Can you work these out from the model? Positions are in its coordinate system, mm. Coordinates: 2 decimals unless noted, no trailing zeros. Loops run counter-clockwise (first coordinate to the right, second up) from the corner with the lowest first, then second, coordinate; pieces in that order, holes last.
```python
from build123d import *

# Parameters (mm, degrees)
SKETCH1_W           = 6
SKETCH1_H           = 50
SKETCH1_W_2         = 50
SKETCH1_H_2         = 6
BOSS_EXTRUDE1_DEPTH = 6


with BuildPart() as part:
    # Sketch1 → Boss-Extrude1 (new body)
    with BuildSketch(Plane(origin=(0, 0, 0), x_dir=(0, 0, -1), z_dir=(1, 0, 0))):
        with BuildLine():
            Line((-396.831767264, 351.151199882), (21.168232736, 351.151199882))
            ThreePointArc((21.168232736, 351.151199882), (91.878910855, 321.861878001), (121.168232736, 251.151199882))
            Line((121.168232736, 251.151199882), (121.168232736, -330.848800118))
            Line((121.168232736, -330.848800118), (-396.831767264, -330.848800118))
            Line((-396.831767264, -330.848800118), (-396.831767264, 351.151199882))
        make_face()
        with Locations((-375.831767264, 251.151199882)):
            Rectangle(SKETCH1_W, SKETCH1_H, mode=Mode.SUBTRACT)
        with Locations((-375.831767264, -230.848800118)):
            Rectangle(SKETCH1_W, SKETCH1_H, mode=Mode.SUBTRACT)
        with Locations((-235.831767264, -309.848800118)):
            Rectangle(SKETCH1_W_2, SKETCH1_H_2, mode=Mode.SUBTRACT)
        with Locations((-39.831767264, -309.848800118)):
            Rectangle(SKETCH1_W_2, SKETCH1_H_2, mode=Mode.SUBTRACT)
        with Locations((-235.831767264, -219.848800118)):
            Rectangle(SKETCH1_W_2, SKETCH1_H_2, mode=Mode.SUBTRACT)
        with Locations((-39.831767264, -219.848800118)):
            Rectangle(SKETCH1_W_2, SKETCH1_H_2, mode=Mode.SUBTRACT)
        with Locations((-235.831767264, -129.848800118)):
            Rectangle(SKETCH1_W_2, SKETCH1_H_2, mode=Mode.SUBTRACT)
        with Locations((-39.831767264, -129.848800118)):
            Rectangle(SKETCH1_W_2, SKETCH1_H_2, mode=Mode.SUBTRACT)
        with Locations((-235.831767264, -39.848800118)):
            Rectangle(SKETCH1_W_2, SKETCH1_H_2, mode=Mode.SUBTRACT)
        with Locations((-39.831767264, -39.848800118)):
            Rectangle(SKETCH1_W_2, SKETCH1_H_2, mode=Mode.SUBTRACT)
        with Locations((-267.331767264, 308.151199882)):
            Rectangle(SKETCH1_W, SKETCH1_H, mode=Mode.SUBTRACT)
        with Locations((-137.831767264, 308.151199882)):
            Rectangle(SKETCH1_W, SKETCH1_H, mode=Mode.SUBTRACT)
    extrude(amount=BOSS_EXTRUDE1_DEPTH)


solid = part.part
```
Item 1: Suppose I cut it at B-B, the plane x = 1. Count the separate pieces of the cut face and the enclosed holes in it, plus the area to 3 significant figures.
Results are:
separate pieces: 1
enclosed holes: 12
area: 348,000 mm2
Item 2: Suppose I cut it at A-A, the plane z = 222.5. Please give me the cut outline in (x, y), plus the area to 3 significant figures.
Results are:
outline: (0, -330.85) - (6, -330.85) - (6, -312.85) - (0, -312.85) - close; (0, -306.85) - (6, -306.85) - (6, -222.85) - (0, -222.85) - close; (0, -216.85) - (6, -216.85) - (6, -132.85) - (0, -132.85) - close; (0, -126.85) - (6, -126.85) - (6, -42.85) - (0, -42.85) - close; (0, -36.85) - (6, -36.85) - (6, 351.15) - (0, 351.15) - close
area: 3,950 mm2
Item 3: I need wall thicknesses on line 1 along Y through (x, z) = (5.4, 34); line 2 along Z through (x, y) = (4.7, 229); line 3 along Y through (x, z) = (4.7, 140). Which ranges of each line are inside material? Lowest first, please.
Results are:
line 1: y = -330.85 to -312.85, -306.85 to -222.85, -216.85 to -132.85, -126.85 to -42.85, -36.85 to 351.15
line 2: z = -121.17 to 372.83, 378.83 to 396.83
line 3: y = -330.85 to 283.15, 333.15 to 351.15
